from build123d import *

# Parameters (mm, degrees)
SKETCH1_R           = 4
SKETCH1_R_2         = 3
BOSS_EXTRUDE1_DEPTH = 19.05
SKETCH2_R           = 7.5
CUT_EXTRUDE1_DEPTH  = 8


with BuildPart() as part:
    # Sketch1 → Boss-Extrude1 (new body)
    with BuildSketch(Plane(origin=(0, 0, 0), x_dir=(1, 0, 0), z_dir=(0, 1, 0))):
        with BuildLine():
            Line((-43, -45), (43, -45))
            ThreePointArc((43, -45), (44.414213562, -44.414213562), (45, -43))
            Line((45, -43), (45, 43))
            ThreePointArc((45, 43), (44.414213562, 44.414213562), (43, 45))
            Line((43, 45), (-43, 45))
            ThreePointArc((-43, 45), (-44.414213562, 44.414213562), (-45, 43))
            Line((-45, 43), (-45, -43))
            ThreePointArc((-45, -43), (-44.414213562, -44.414213562), (-43, -45))
        make_face()
        with Locations((-32.5, 32.5)):
            Circle(SKETCH1_R, mode=Mode.SUBTRACT)
        with Locations((32.5, 32.5)):
            Circle(SKETCH1_R, mode=Mode.SUBTRACT)
        with Locations((32.5, -32.5)):
            Circle(SKETCH1_R, mode=Mode.SUBTRACT)
        with Locations((-32.5, -32.5)):
            Circle(SKETCH1_R, mode=Mode.SUBTRACT)
        with Locations((-32.5, 0)):
            Circle(SKETCH1_R_2, mode=Mode.SUBTRACT)
        with Locations((32.5, 0)):
            Circle(SKETCH1_R_2, mode=Mode.SUBTRACT)
    extrude(amount=BOSS_EXTRUDE1_DEPTH)

    # Sketch2 → Cut-Extrude1 (cut)
    with BuildSketch(Plane(origin=(0, 19.05, 0), x_dir=(1, 0, 0), z_dir=(0, 1, 0))):
        with Locations((-32.5, -32.5)):
            Circle(SKETCH2_R)
        with Locations((32.5, -32.5)):
            Circle(SKETCH2_R)
        with Locations((32.5, 32.5)):
            Circle(SKETCH2_R)
        with Locations((-32.5, 32.5)):
            Circle(SKETCH2_R)
    extrude(amount=-CUT_EXTRUDE1_DEPTH, mode=Mode.SUBTRACT)


solid = part.part
Verification items for the finished model (mm, model axes). A direction names the side the tool comes from. Coordinates: 2 decimals unless noted, no trailing zeros. Order: outer loops, then holes, each group sorted by start corner. A loop starts at its lowest first (then second) coordinate and runs counter-clockwise, first axis right, second up. Notation, with made-up numbers: (-6.75, -34.75) -> (18.25, -34.75) arc R17 cw to (18.25, -16.75) -> close; hole circle Ø6 at (-12.5, 15.5). An arc over 180 degrees is marked (long way). Put each result on its own line as item: value. Start each with the question number.
1. Access from +Z, -Z, +X, -X, +Y, -Y to the whole of each face (thin tool, end or side, straight path). Record for faces 4 (the cylindrical face through (29.5, 9.4, -0.1)), 5 (the flat face through (36, 11.05, 36)).
2. Cross-section at A-A, the plane z = 32.5. Record the boundary of the cut face in (x, y), then the cut area to 3 significant figures.
3. Go/stop test with a flat-tipped pin: pin 1 Ø4.5 at (x, z) = (35.5, -32) entering from +Y. Record where the tip stops, or that it passes through.
4. Cross-section at D-D, the plane x = -38. Record the boundary of the cut face in (y, z).
5. Material ranges on L1, parallel to X at y = 16, z = -32.5; L2, parallel to X at y = 6.5, z = -32.5; L3, parallel to Z at x = -32.5, y = 4, recorded low to high. Write a range as [from, to].
6. Mould release check, pull along Z, two halves, no side actions. Record for faces 1 (the cylindrical face through (-44.43, 9.39, 44.4)), 2 (the cylindrical face through (-44.4, 9.39, -44.43)), 3 (the cylindrical face through (30.87, 15.11, 39.82)): released by +Z, released by -Z, zero draft, split by the parting line, or undercut.
7. Cross-section at C-C, the plane y = 5.5. Record the boundary of the cut face in (x, z), then the cut area to 3 significant figures.
8. Cross-section at B-B, the plane x = 32.5. Record the boundary of the cut face in (y, z).
Computed:
1. face 4: +Y, -Y
1. face 5: +Y
2. outline: (-45, 0) -> (-36.5, 0) -> (-36.5, 11.05) -> (-40, 11.05) -> (-40, 19.05) -> (-45, 19.05) -> close; (-28.5, 0) -> (28.5, 0) -> (28.5, 11.05) -> (25, 11.05) -> (25, 19.05) -> (-25, 19.05) -> (-25, 11.05) -> (-28.5, 11.05) -> close; (36.5, 0) -> (45, 0) -> (45, 19.05) -> (40, 19.05) -> (40, 11.05) -> (36.5, 11.05) -> close
2. area: 1,300 mm2
3. pin 1: y = 11.05
4. outline: (0, -45) -> (19.05, -45) -> (19.05, -37.6) -> (11.05, -37.6) -> (11.05, -27.4) -> (19.05, -27.4) -> (19.05, 27.4) -> (11.05, 27.4) -> (11.05, 37.6) -> (19.05, 37.6) -> (19.05, 45) -> (0, 45) -> close
5. L1: [-45, -40], [-25, 25], [40, 45]
5. L2: [-45, -36.5], [-28.5, 28.5], [36.5, 45]
5. L3: [-45, -36.5], [-28.5, -3], [3, 28.5], [36.5, 45]
6. face 1: released by +Z
6. face 2: released by -Z
6. face 3: undercut
7. outline: (-45, -43) arc R2 ccw to (-43, -45) -> (43, -45) arc R2 ccw to (45, -43) -> (45, 43) arc R2 ccw to (43, 45) -> (-43, 45) arc R2 ccw to (-45, 43) -> close; hole circle Ø8 at (-32.5, -32.5); hole circle Ø8 at (-32.5, 32.5); hole circle Ø6 at (-32.5, 0); hole circle Ø8 at (32.5, -32.5); hole circle Ø8 at (32.5, 32.5); hole circle Ø6 at (32.5, 0)
7. area: 7,840 mm2
8. outline: (0, -45) -> (19.05, -45) -> (19.05, -40) -> (11.05, -40) -> (11.05, -36.5) -> (0, -36.5) -> close; (0, -28.5) -> (11.05, -28.5) -> (11.05, -25) -> (19.05, -25) -> (19.05, -3) -> (0, -3) -> close; (0, 3) -> (19.05, 3) -> (19.05, 25) -> (11.05, 25) -> (11.05, 28.5) -> (0, 28.5) -> close; (0, 36.5) -> (11.05, 36.5) -> (11.05, 40) -> (19.05, 40) -> (19.05, 45) -> (0, 45) -> close
